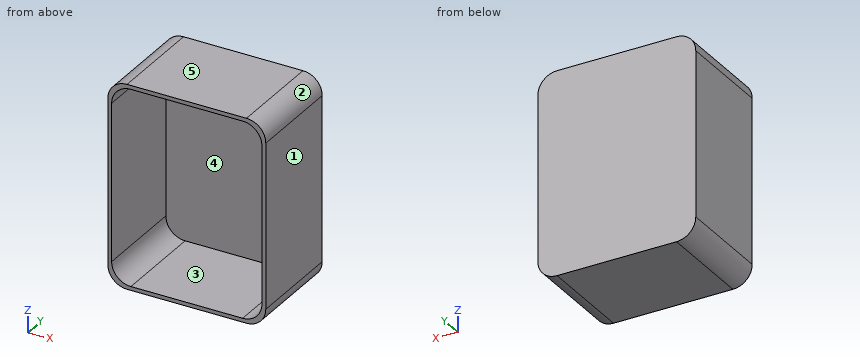
```python
from build123d import *

# Parameters (mm, degrees)
BOX016_W     = 78
BOX016_H     = 50.5
BOX016_DEPTH = 101.5
FILLET018_R  = 10
BOX015_W     = 82
BOX015_H     = 50.5
BOX015_DEPTH = 105.5
FILLET015_R  = 10


with BuildPart() as innerboxcut001:
    # Box016 → Box016 (new body)
    with BuildSketch(Plane(origin=(78, 24, -13.75), x_dir=(-1, 0, 0), z_dir=(0, 0, 1))):
        with Locations((39, 25.25)):
            Rectangle(BOX016_W, BOX016_H)
    extrude(amount=BOX016_DEPTH)

    # Fillet018
    fillet018_edges = [innerboxcut001.edges().sort_by_distance(p)[0] for p in [
        (78, -1.25, 87.75),
        (78, -1.25, -13.75),
        (0, -1.25, 87.75),
        (0, -1.25, -13.75),
    ]]
    fillet(fillet018_edges, radius=FILLET018_R)


with BuildPart() as outershellbottom:
    # Box015 → Box015 (new body)
    with BuildSketch(Plane(origin=(80, 26, -15.75), x_dir=(-1, 0, 0), z_dir=(0, 0, 1))):
        with Locations((41, 25.25)):
            Rectangle(BOX015_W, BOX015_H)
    extrude(amount=BOX015_DEPTH)

    # Fillet015
    fillet015_edges = [outershellbottom.edges().sort_by_distance(p)[0] for p in [
        (80, 0.75, 89.75),
        (80, 0.75, -15.75),
        (-2, 0.75, 89.75),
        (-2, 0.75, -15.75),
    ]]
    fillet(fillet015_edges, radius=FILLET015_R)

    # Cut006: cut innerBoxCut001
    add(innerboxcut001.part, mode=Mode.SUBTRACT)


solid = outershellbottom.part
```
Model file for the job. Use its own axes, mm. Face numbers are marked on the shaded views. A direction names the side the tool comes from. Give positions to 0.01 mm unless a question says otherwise; leave off trailing zeros. Write each loop counter-clockwise with the first axis right and the second up, starting at its lowest first coordinate (ties: lowest second). Pieces come first, ordered by that corner, then holes. Notation, with made-up numbers: (68, -25) - (125, -25) arc R24 cw to (125, 13) - close; hole circle Ø6 at (39.25, 17). An arc over 180 degrees is marked (long way). One line per question, with ' | ' between items. Start each with the question number.
(1) Slice it at C-C on z = 53.5. Write the cut outline in (x, y).
(2) Two-plate mould, pull along Z, no slides. Class the marked faces 1, 2 and 3: +Z half, -Z half, draft (parallel to the pull), parting line (faces both ways), or undercut.
(3) Slice it at A-A on y = -20.5. Write the cut outline in (x, z).
(4) Wall check: line 1 along Z through (x, y) = (58.5, -7.5); line 2 along X through (y, z) = (8.5, 71.5). Give the ranges that are in metal, low to high. Write a range as from..to.
(5) Slice it at B-B on x = 18. Write the cut outline in (y, z).
(6) 3-axis set-ups, long thin cutter, end or side, ignore diameter. For the marked faces 4 and 5: which of +Z, -Z, +X, -X, +Y, -Y reach the whole face in a straight line?
Results below:
1) outline: (-2, -24.5) - (0, -24.5) - (0, 24) - (78, 24) - (78, -24.5) - (80, -24.5) - (80, 26) - (-2, 26) - close
2) face 1: draft | face 2: +Z half | face 3: undercut
3) outline: (-2, -5.75) arc R10 ccw to (8, -15.75) - (70, -15.75) arc R10 ccw to (80, -5.75) - (80, 79.75) arc R10 ccw to (70, 89.75) - (8, 89.75) arc R10 ccw to (-2, 79.75) - close; hole (0, -3.75) arc R10 ccw to (10, -13.75) - (68, -13.75) arc R10 ccw to (78, -3.75) - (78, 77.75) arc R10 ccw to (68, 87.75) - (10, 87.75) arc R10 ccw to (0, 77.75) - close
4) line 1: -15.75..-13.75, 87.75..89.75 | line 2: -2..0, 78..80
5) outline: (-24.5, -15.75) - (26, -15.75) - (26, 89.75) - (-24.5, 89.75) - (-24.5, 87.75) - (24, 87.75) - (24, -13.75) - (-24.5, -13.75) - close
6) face 4: -Y | face 5: +Z, +X, -X, +Y, -Y
